from build123d import *

# Parameters (mm, degrees)
SKETCH1_R           = 2
BOSS_EXTRUDE1_DEPTH = 5
SKETCH3_R           = 1
BOSS_EXTRUDE2_DEPTH = 4
BOSS_EXTRUDE3_DEPTH = 2
CHAMFER1_SIZE       = 0.5


with BuildPart() as part:
    # Sketch1 → Boss-Extrude1 (new body)
    with BuildSketch(Plane(origin=(0, 0, 0), x_dir=(0, 0, -1), z_dir=(1, 0, 0))):
        Circle(SKETCH1_R)
    extrude(amount=BOSS_EXTRUDE1_DEPTH)

    # Sketch3 → Boss-Extrude2 (add)
    with BuildSketch(Plane(origin=(5, 0, 0), x_dir=(0, 0, -1), z_dir=(1, 0, 0))):
        Circle(SKETCH3_R)
    extrude(amount=BOSS_EXTRUDE2_DEPTH)

    # Sketch4 → Boss-Extrude3 (add)
    with BuildSketch(Plane(origin=(9, 0, 0), x_dir=(0, 0, -1), z_dir=(1, 0, 0))):
        Polygon((0, -2.886751346), (2.5, -1.443375673), (2.5, 1.443375673), (0, 2.886751346), (-2.5, 1.443375673), (-2.5, -1.443375673), align=None)
    extrude(amount=BOSS_EXTRUDE3_DEPTH)

    # Chamfer1
    chamfer1_edges = [part.edges().sort_by_distance(p)[0] for p in [
        (0, 0, 2),
    ]]
    chamfer(chamfer1_edges, length=CHAMFER1_SIZE)


solid = part.part
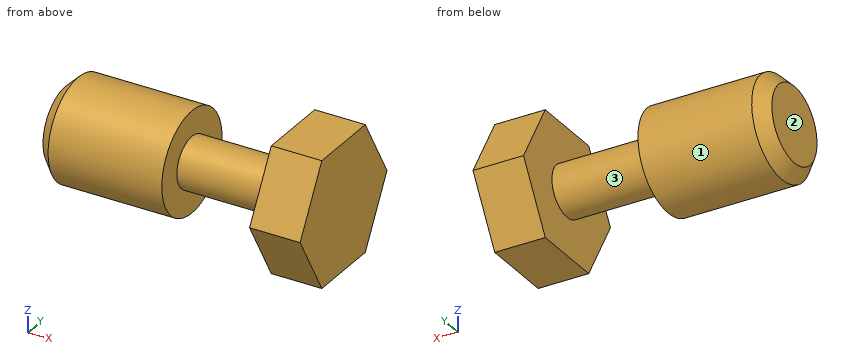
Can you work these out from the model? Positions are in its coordinate system, mm. Face numbers are marked on the shaded views. A direction names the side the tool comes from. Give positions to 0.01 mm unless a question says otherwise; leave off trailing zeros. Loops run counter-clockwise (first coordinate to the right, second up) from the corner with the lowest first, then second, coordinate; pieces in that order, holes last. Notation, with made-up numbers: (36.5, 33.5) - (77.5, 33.5) arc R18 ccw to (77.5, 65.5) - close; hole circle Ø3 at (47.5, 4). An arc over 180 degrees is marked (long way). One line per item, written item: value.
(1) I need wall thicknesses on line 1 along X through (y, z) = (-1, -0.5); line 2 along X through (y, z) = (2.1, -0.5); line 3 along X through (y, z) = (-1.6, -1.05). Which ranges of each line are inside material? Lowest first, please.
Verdict:
line 1: 0 to 5, 9 to 11
line 2: 9 to 11
line 3: 0.41 to 5, 9 to 11
(2) If we section it at B-B, the plane x = 1.25: List the corners of the cut face in (y, z) for me, plus the area to 3 significant figures.
Verdict:
outline: circle Ø4 at (0, 0)
area: 12.6 mm^2
(3) On a 3-axis mill with a long thin cutter (end or side, diameter ignored), from which of +Z, -Z, +X, -X, +Y, -Y can I reach the whole of each face in a straight line? I mean the marked faces 1, 2 and 3. Say none if no direction works.
Verdict:
face 1: -X
face 2: +Z, -Z, -X, +Y, -Y
face 3: none
(4) If we section it at A-A, the plane y = 0: List the corners of the cut face in (x, z) for me.
Verdict:
outline: (0, -1.5) - (0.5, -2) - (5, -2) - (5, -1) - (9, -1) - (9, -2.5) - (11, -2.5) - (11, 2.5) - (9, 2.5) - (9, 1) - (5, 1) - (5, 2) - (0.5, 2) - (0, 1.5) - close
(5) I'm going to push flat-ended pins straight in: pin 1 (2 mm diameter, centred on x = 4.5, z = -1.5, fed in from -Y); pin 2 (3 mm diameter, centred on x = 1.5, y = -1.5, fed in from +Z). Where does each tip first touch, or does it pass through?
Verdict:
pin 1: y = -1.94
pin 2: z = 2
(6) If we section it at C-C, the plane x = 5.25: List the corners of the cut face in (y, z) for me, plus the area to 3 significant figures.
Verdict:
outline: circle Ø2 at (0, 0)
area: 3.14 mm^2
